Check sheet for the modelled part. Datum: model origin and axes. Units: mm. A direction names the side the tool comes from. Give positions to 0.01 mm unless a question says otherwise; leave off trailing zeros. Order: outer loops, then holes, each group sorted by start corner. A loop starts at its lowest first (then second) coordinate and runs counter-clockwise, first axis right, second up. Notation, with made-up numbers: M -38.5,-33.75 L -5.5,-33.75 A33 ccw -5.5,-0.75 Z; hole C 83,-3.75 d1. An arc over 180 degrees is marked long. Answer in a Markdown table with one row per item. Add a question column.
Autodesk Inventor part; units mm, degrees
ref_plane "YZ Plane" through (0, 0, 0) normal (1, 0, 0) x (0, 1, 0)
ref_plane "XZ Plane" through (0, 0, 0) normal (0, 1, 0) x (-1, 0, 0)
ref_plane "XY Plane" through (0, 0, 0) normal (0, 0, 1) x (1, 0, 0)
sketch "Sketch1" plane through (0, 0, 0) normal (0, 0, 1) x (1, 0, 0)
  line L0 (0, 0) -> (42, 0)
  line L1 (42, 0) -> (42, 42)
  line L2 (42, 42) -> (0, 42)
  line L3 (0, 42) -> (0, 0)
  dimension "d0" = 42
  dimension "d1" = 42
extrude "Extrusion1" add sketch "Sketch1" along normal blind 47
chamfer "Chamfer1" distance 3.5 angle 45 4 edges at (0, 42, 23.5) (0, 0, 23.5) (42, 0, 23.5) (42, 42, 23.5)
sketch "Sketch2" plane through (0, 0, 47) normal (0, 0, 1) x (1, 0, 0)
  circle A0 centre (21, 21) radius 11
  point P0 (0, 0)
  dimension "d7" = 22
extrude "Extrusion2" add sketch "Sketch2" along normal blind 2
sketch "Sketch3" plane through (21, 21, 49) normal (0, 0, 1) x (1, 0, 0)
  circle A0 centre (0, 0) radius 11
  circle A1 centre (0, 0) radius 2.5
  point P0 (-21, -21)
  dimension "d10" = 5
extrude "Extrusion3" add sketch "Sketch3" along normal blind 22 contours A1
sketch "Sketch4" plane through (0, 0, 47) normal (0, 0, 1) x (1, 0, 0)
  line L0 (0, 38.5) -> (0, 3.5)
  line L1 (3.5, 0) -> (38.5, 0)
  circle A0 centre (5.5, 36.5) radius 1.5
  circle A1 centre (36.5, 36.5) radius 1.5
  circle A2 centre (36.5, 5.5) radius 1.5
  circle A3 centre (5.5, 5.5) radius 1.5
  point P0 (0, 0)
  dimension "d13" = 3
  dimension "d14" = 3
  dimension "d15" = 3
  dimension "d16" = 3
  dimension "d17" = 31
  dimension "d18" = 31
  dimension "d19" = 31
  dimension "d20" = 31
  dimension "d21" = 5.5
  dimension "d22" = 5.5
extrude "Extrusion4" cut sketch "Sketch4" against normal blind 4.5
properties part number "NEMA17StepperMotor"
Q1. Draft check along X on faces 3 (the flat face through (5, 6, 42.5)), 4 (the flat face through (21, 21, 71)), 5 (the flat face through (40.3, 40.2, 23.2)). Enter one of: pulls with the +X half, pulls with the -X half, needs draft (parallel to the pull), parting line crosses it, or undercut.
Q2. Thickness scan on probe 1 along Y at (x, z) = (36, 44); probe 2 along Z at (x, y) = (31, 9.5); probe 3 along Z at (x, y) = (16, 28). Record the ranges inside material, lowest first.
Q3. Cross-section at D-D (z = 63). Record the boundary of the cut face in (x, y).
Q4. Go/stop test with flat-tipped pins: pin 1 (4 mm diameter, centred on x = 5.5, y = 5.5, fed in from +Z); pin 2 (1.5 mm diameter, centred on x = 36.5, y = 5.5, fed in from +Z); pin 3 (2 mm diameter, centred on x = 18.5, z = 55.5, fed in from -Y). Record where each tip stops, or that it passes through.
Q5. Cross-section at A-A (y = 36.5). Record the boundary of the cut face in (x, z).
Q6. Tool access check on faces 1 (the flat face through (5, 37, 42.5)), 2 (the flat face through (0, 21, 23)). Record the directions out of +Z, -Z, +X, -X, +Y, -Y that give a thin tool (end or side, any length) a straight path to the whole face; none if there is none.
Q7. Cross-section at C-C (z = 46). Record the boundary of the cut face in (x, y).
Q8. Cross-section at B-B (x = 21). Record the boundary of the cut face in (y, z), and give its area (3 significant figures).
Values follow:
| question | item | result |
|---|---|---|
| 1 | face 3 | undercut |
| 1 | face 4 | needs draft |
| 1 | face 5 | pulls with the +X half |
| 2 | probe 1 | 0 to 4.09, 6.91 to 35.09, 37.91 to 42 |
| 2 | probe 2 | 0 to 47 |
| 2 | probe 3 | 0 to 49 |
| 3 | outline | C 21,21 d5 |
| 4 | pin 1 | z = 47 |
| 4 | pin 2 | z = 42.5 |
| 4 | pin 3 | y = 19 |
| 5 | outline | M 0,0 L 42,0 L 42,47 L 38,47 L 38,42.5 L 35,42.5 L 35,47 L 7,47 L 7,42.5 L 4,42.5 L 4,47 L 0,47 Z |
| 6 | face 1 | +Z |
| 6 | face 2 | +Z, -Z, -X, +Y, -Y |
| 7 | outline | M 0,3.5 L 3.5,0 L 38.5,0 L 42,3.5 L 42,38.5 L 38.5,42 L 3.5,42 L 0,38.5 Z; hole C 5.5,5.5 d3; hole C 5.5,36.5 d3; hole C 36.5,5.5 d3; hole C 36.5,36.5 d3 |
| 8 | outline | M 0,0 L 42,0 L 42,47 L 32,47 L 32,49 L 23.5,49 L 23.5,71 L 18.5,71 L 18.5,49 L 10,49 L 10,47 L 0,47 Z |
| 8 | area | 2,130 mm² |
